Here's how the part is built. I have some questions about the finished solid (model axes, mm). A direction names the side the tool comes from. Round coordinates to 2 decimals unless told otherwise and drop trailing zeros. Order: outer loops, then holes, each group sorted by start corner. A loop starts at its lowest first (then second) coordinate and runs counter-clockwise, first axis right, second up. Notation, with made-up numbers: M 64,38 L 109,38 A15 ccw 109,47 Z; hole C 20,47.5 d5. An arc over 180 degrees is marked long. Write item = value, one per line. Start each with the question number.
Item 1: Please list where these lines run through material, in increasing order: L1, parallel to Y at x = -45, z = 4; L2, parallel to Z at x = 0.5, y = 99.5; L3, parallel to Z at x = -1.5, y = 10.
Item 2: I want a section at A-A, the plane x = 21. List the corners of the cut face in (y, z) for me, plus the area to 3 significant figures.
Item 3: I want a section at C-C, the plane y = -5. List the corners of the cut face in (x, z) for me, plus the area to 3 significant figures.
Item 4: I want a section at B-B, the plane z = -17. List the corners of the cut face in (x, y) for me, plus the area to 3 significant figures.
Item 5: I'm going to push flat-ended pins straight in: P1, Ø1.5, axis at x = -22, z = 29.5, coming from the +Y side; P2, Ø10, axis at y = 77, z = 20, coming from the -X side; P3, Ø1.7, axis at x = 3, z = 23, coming from the +Y side; P4, Ø4, axis at x = 18, z = 13.5, coming from the +Y side. Where does each tip first touch, or does it pass through?
Item 6: For faces 4 (the face through (0, 185, 21.651)), 5 (the face through (-23.846, 114.79, 7.509)), 6 (the face through (20, 170, -12)), which set-ups out of +Z, -Z, +X, -X, +Y, -Y let a thin tool reach every point of the face, with its end or its side?
Item 7: We'd pull the mould along Y, two halves only. Please class faces 1 (the face through (-20, 170, -12)), 2 (the face through (11.5, 50, 5.9)), 3 (the face through (22, -71, -14.246)): pulls with the +Y half, pulls with the -Y half, needs draft (parallel to the pull), parting line crosses it, or undercut.
Item 8: I want a section at D-D, the plane x = 43.5. List the corners of the cut face in (y, z) for me, plus the area to 3 significant figures.
```python
from build123d import *

# Parameters (mm, degrees)
F0_R          = 50
F1_DEPTH      = 100
F2_R          = 25
F3_DEPTH      = 50
F4_R          = 12.5
F5_DEPTH      = 10
F6_R          = 25
F7_DEPTH      = 30
F8_R          = 12.5
F9_DEPTH      = 10
F10_R         = 25
F11_DEPTH     = 30
F12_R         = 12.5
F13_DEPTH     = 10
F14_R         = 25
F15_DEPTH     = 30
F17_DEPTH     = 30
F20_D         = 70
F22_DEPTH     = 75
F23_T4_DEPTH  = 295.3549985752
F23_S5_R      = 50
F23_T6_DEPTH  = 152
F23_T10_DEPTH = 295.3549985752
F23_S11_R     = 50
F23_T12_DEPTH = 152


# Not quite as in the source:
# - a fillet or chamfer that OpenCascade refuses, or shapes differently, is made with other operations: its cross-section is extruded or revolved along the edge and cut away or added


with BuildPart() as f1:
    # F0 (on Front) → F1 (new body)
    with BuildSketch(Plane.XZ):
        Circle(F0_R)
    extrude(amount=F1_DEPTH)

    # F2 (on face) → F3 (join)
    with BuildSketch(Plane(origin=(0, 0, 0), x_dir=(-1, 0, 0), z_dir=(0, 1, 0))):
        Circle(F2_R)
    extrude(amount=F3_DEPTH)

    # F4 (on face) → F5 (join)
    with BuildSketch(Plane(origin=(0, 50, 0), x_dir=(-1, 0, 0), z_dir=(0, 1, 0))):
        Circle(F4_R)
    extrude(amount=F5_DEPTH)

    # F6 (on face) → F7 (join)
    with BuildSketch(Plane(origin=(0, 60, 0), x_dir=(-1, 0, 0), z_dir=(0, 1, 0))):
        Circle(F6_R)
    extrude(amount=F7_DEPTH)

    # F8 (on face) → F9 (join)
    with BuildSketch(Plane(origin=(0, 90, 0), x_dir=(-1, 0, 0), z_dir=(0, 1, 0))):
        Circle(F8_R)
    extrude(amount=F9_DEPTH)

    # F10 (on face) → F11 (join)
    with BuildSketch(Plane(origin=(0, 100, 0), x_dir=(-1, 0, 0), z_dir=(0, 1, 0))):
        Circle(F10_R)
    extrude(amount=F11_DEPTH)

    # F12 (on face) → F13 (join)
    with BuildSketch(Plane(origin=(0, 130, 0), x_dir=(-1, 0, 0), z_dir=(0, 1, 0))):
        Circle(F12_R)
    extrude(amount=F13_DEPTH)

    # F14 (on face) → F15 (join)
    with BuildSketch(Plane(origin=(0, 140, 0), x_dir=(-1, 0, 0), z_dir=(0, 1, 0))):
        Circle(F14_R)
    extrude(amount=F15_DEPTH)

    # F16 (on face) → F17 (join)
    with BuildSketch(Plane(origin=(0, 170, 0), x_dir=(-1, 0, 0), z_dir=(0, 1, 0))):
        Polygon((12.5, -21.6506350946), (25, 0), (12.5, 21.6506350946), (-12.5, 21.6506350946), (-25, 0), (-12.5, -21.6506350946), align=None)
    extrude(amount=F17_DEPTH)

    # F20 (through all)
    with Locations(Plane.XY.offset(50)):
        with Locations((0, -99.9434366822)):
            Hole(F20_D / 2)

    # F21 (on face) → F22 (cut)
    with BuildSketch(Plane.XZ.offset(100)):
        with BuildLine():
            ThreePointArc((47.9274992876, 14.2462209739), (0, 50), (-47.9274992876, 14.2462209739))
            Line((-47.9274992876, 14.2462209739), (47.9274992876, 14.2462209739))
        make_face()
        with BuildLine():
            Line((47.9274992876, -14.2462209739), (-47.9274992876, -14.2462209739))
            ThreePointArc((-47.9274992876, -14.2462209739), (0, -50), (47.9274992876, -14.2462209739))
        make_face()
    extrude(amount=-F22_DEPTH, mode=Mode.SUBTRACT)

    # F23: fillet of radius 39.9 on 2 edges, made by hand


with BuildPart() as f23_tool2:
    # F23_s3 → F23_t4 (new body)
    with BuildSketch(Plane.YZ.offset(-147.6774992876)):
        with BuildLine():
            ThreePointArc((-64.9, 14.2462209739), (-36.6864394307, 25.9326604046), (-25, 54.1462209739))
            Line((-25, 54.1462209739), (-25, 14.2462209739))
            Line((-25, 14.2462209739), (-64.9, 14.2462209739))
        make_face()
    extrude(amount=F23_T4_DEPTH)

    # F23_s5 → F23_t6 (intersect, symmetric)
    with BuildSketch(Plane.XZ.offset(44.9)):
        Circle(F23_S5_R)
    extrude(amount=F23_T6_DEPTH, both=True, mode=Mode.INTERSECT)


with BuildPart() as f1_1:
    add(f1.part)

    # F23_t1: union F23_tool2
    add(f23_tool2.part)


with BuildPart() as f23_tool8:
    # F23_s9 → F23_t10 (new body)
    with BuildSketch(Plane.YZ.offset(147.6774992876)):
        with BuildLine():
            ThreePointArc((-64.9, -14.2462209739), (-36.6864394307, -25.9326604046), (-25, -54.1462209739))
            Line((-25, -54.1462209739), (-25, -14.2462209739))
            Line((-25, -14.2462209739), (-64.9, -14.2462209739))
        make_face()
    extrude(amount=-F23_T10_DEPTH)

    # F23_s11 → F23_t12 (intersect, symmetric)
    with BuildSketch(Plane.XZ.offset(44.9)):
        Circle(F23_S11_R)
    extrude(amount=F23_T12_DEPTH, both=True, mode=Mode.INTERSECT)


with BuildPart() as f1_2:
    add(f1_1.part)

    # F23_t7: union F23_tool8
    add(f23_tool8.part)


solid = f1_2.part
```
Filled in:
q1.L1 = -100 to 0
q1.L2 = -12.49 to 12.49
q1.L3 = -24.95 to 24.95
q2.outline = M -71.94,-14.25 L -64.9,-14.25 A39.9 cw -25.98,-45.38 L 0,-45.38 L 0,-13.56 L 50,-13.56 L 50,13.56 L 0,13.56 L 0,45.38 L -25.98,45.38 A39.9 cw -64.9,14.25 L -71.94,14.25 Z; M 60,-13.56 L 90,-13.56 L 90,13.56 L 60,13.56 Z; M 100,-13.56 L 130,-13.56 L 130,13.56 L 100,13.56 Z; M 140,-13.56 L 170,-13.56 L 170,-6.93 L 200,-6.93 L 200,6.93 L 170,6.93 L 170,13.56 L 140,13.56 Z
q2.area = 8,500 mm^2
q3.outline = C 0,0 d100
q3.area = 7,850 mm^2
q4.outline = M -47.02,-50.33 L 47.02,-50.33 L 47.02,0 L 18.33,0 L 18.33,50 L -18.33,50 L -18.33,0 L -47.02,0 Z; M -18.33,60 L 18.33,60 L 18.33,90 L -18.33,90 Z; M -18.33,100 L 18.33,100 L 18.33,130 L -18.33,130 Z; M -18.33,140 L 18.33,140 L 18.33,170 L 15.19,170 L 15.19,200 L -15.19,200 L -15.19,170 L -18.33,170 Z
q4.area = 10,800 mm^2
q5.P1 = 0
q5.P2 = -20
q5.P3 = 170
q5.P4 = 200
q6.face_4 = +Z, +X, -X, +Y
q6.face_5 = +Y
q6.face_6 = -Z, +X, +Y
q7.face_1 = pulls with the +Y half
q7.face_2 = undercut
q7.face_3 = needs draft
q8.outline = M -100,-14.25 L -64.9,-14.25 A39.9 cw -38.03,-24.65 L 0,-24.65 L 0,24.65 L -38.03,24.65 A39.9 cw -64.9,14.25 L -100,14.25 Z
q8.area = 3,820 mm^2
